Here's how the part is built. I have some questions about the finished solid (model axes, mm). Face numbers are marked on the shaded views. A direction names the side the tool comes from. Give positions to 0.01 mm unless a question says otherwise; leave off trailing zeros. Loops run counter-clockwise (first coordinate to the right, second up) from the corner with the lowest first, then second, coordinate; pieces in that order, holes last. Notation, with made-up numbers: (49.5, 2.5) - (104.5, 2.5) arc R16 cw to (104.5, 12.5) - close; hole circle Ø4 at (3.25, 49.5). An arc over 180 degrees is marked (long way). Use a Markdown table: item, result.
from build123d import *

# Parameters (mm, degrees)
SKETCH026_R          = 6
PAD012_DEPTH         = 1
SKETCH027_R          = 4
PAD013_DEPTH         = 21
SKETCH028_R          = 2.55
POCKET010_DEPTH      = 1.001
POCKET010_DEPTH_BACK = 21.001
CHAMFER_SIZE2        = 1
CHAMFER_SIZE         = 0.5


with BuildPart() as part:
    # Sketch026 → Pad012 (new body)
    with BuildSketch(Plane.XY):
        Circle(SKETCH026_R)
    extrude(amount=-PAD012_DEPTH)

    # Sketch027 → Pad013 (join)
    with BuildSketch(Plane.XY):
        Circle(SKETCH027_R)
    extrude(amount=PAD013_DEPTH)

    # Sketch028 → Pocket010 (cut, two sides)
    with BuildSketch(Plane.XY) as pocket010_sk:
        Circle(SKETCH028_R)
    extrude(amount=-POCKET010_DEPTH, mode=Mode.SUBTRACT)
    extrude(pocket010_sk.sketch, amount=POCKET010_DEPTH_BACK, mode=Mode.SUBTRACT)

    # Chamfer
    chamfer_edges = [part.edges().sort_by_distance(p)[0] for p in [
        (-2.55, 0, -1),
    ]]
    chamfer_side = part.faces().sort_by_distance((-5.830294, 0, -1))[0]
    chamfer(chamfer_edges, length=CHAMFER_SIZE, length2=CHAMFER_SIZE2, reference=chamfer_side)


solid = part.part
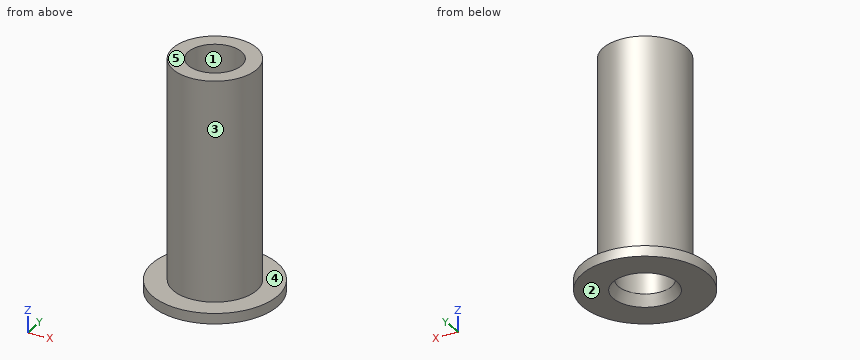
(1) We'd pull the mould along Y, two halves only. Please class the marked faces 1, 2 and 3: pulls with the +Y half, pulls with the -Y half, needs draft (parallel to the pull), parting line crosses it, or undercut.
A:
| item | result |
|---|---|
| face 1 | undercut |
| face 2 | needs draft |
| face 3 | parting line crosses it |
(2) If I drill on line 1 (Y direction, x = 0, z = 15.25); line 2 (X direction, y = 0.25, z = 15); line 3 (Y direction, x = 1, z = 5), over which ranges is the centre line in solid material (lowest first)?
A:
| item | result |
|---|---|
| line 1 | -4 to -2.55, 2.55 to 4 |
| line 2 | -3.99 to -2.54, 2.54 to 3.99 |
| line 3 | -3.87 to -2.35, 2.35 to 3.87 |
(3) Suppose I cut it at C-C on z = 18.75. Write out the boundary of the cut face in (x, y).
A:
| item | result |
|---|---|
| outline | circle Ø8 at (0, 0); hole circle Ø5.1 at (0, 0) |
(4) On a 3-axis mill with a long thin cutter (end or side, diameter ignored), from which of +Z, -Z, +X, -X, +Y, -Y can I reach the whole of each face in a straight line? I mean the marked faces 4 and 5. Say none if no direction works.
A:
| item | result |
|---|---|
| face 4 | +Z |
| face 5 | +Z, +X, -X, +Y, -Y |
(5) Suppose I cut it at D-D on y = 5. Write out the boundary of the cut face in (x, z), plus the area to 3 significant figures.
A:
| item | result |
|---|---|
| outline | (-3.32, -1) - (3.32, -1) - (3.32, 0) - (-3.32, 0) - close |
| area | 6.63 mm2 |
(6) Suppose I cut it at A-A on x = 0. Write out the boundary of the cut face in (y, z).
A:
| item | result |
|---|---|
| outline | (-6, -1) - (-3.05, -1) - (-2.55, 0) - (-2.55, 21) - (-4, 21) - (-4, 0) - (-6, 0) - close; (2.55, 0) - (3.05, -1) - (6, -1) - (6, 0) - (4, 0) - (4, 21) - (2.55, 21) - close |
(7) Will these pins go through, and if not, where does the flat tip stop? pin 1 (2 mm diameter, centred on x = 0.5, z = 5.5, fed in from +Y); pin 2 (4 mm diameter, centred on y = -0.5, z = 12.5, fed in from +X); pin 3 (4 mm diameter, centred on y = 4, z = 2.5, fed in from -X).
A:
| item | result |
|---|---|
| pin 1 | y = 4 |
| pin 2 | x = 4 |
| pin 3 | x = -3.46 |
